For this review, take the finished solid that the model builds, in its own axes (mm). Give positions to 0.01 mm unless a question says otherwise; leave off trailing zeros. Write each loop counter-clockwise with the first axis right and the second up, starting at its lowest first coordinate (ties: lowest second). Pieces come first, ordered by that corner, then holes. Notation, with made-up numbers: M -21,64.25 L 18,64.25 A22 ccw 18,96.25 Z; hole C 81.25,41 d5. An arc over 180 degrees is marked long. Answer as a JSON object with one key per item and string values. Group by question number.
```python
from build123d import *

# Parameters (mm, degrees)
BOSS_EXTRUDE1_DEPTH    = 5
M2_5_CLEARANCE_HOLE1_D = 2.9


with BuildPart() as part:
    # Sketch1 → Boss-Extrude1 (new body)
    with BuildSketch(Plane.XY):
        with BuildLine():
            Line((5, 25), (5, -25))
            ThreePointArc((5, -25), (0, -30), (-5, -25))
            Line((-5, -25), (-5, 25))
            ThreePointArc((-5, 25), (0, 30), (5, 25))
        make_face()
    extrude(amount=BOSS_EXTRUDE1_DEPTH)

    # M2.5 Clearance Hole1 (through all)
    with Locations(Plane.XY.offset(5)):
        with Locations((0, 25), (0, -25)):
            Hole(M2_5_CLEARANCE_HOLE1_D / 2)


solid = part.part
```
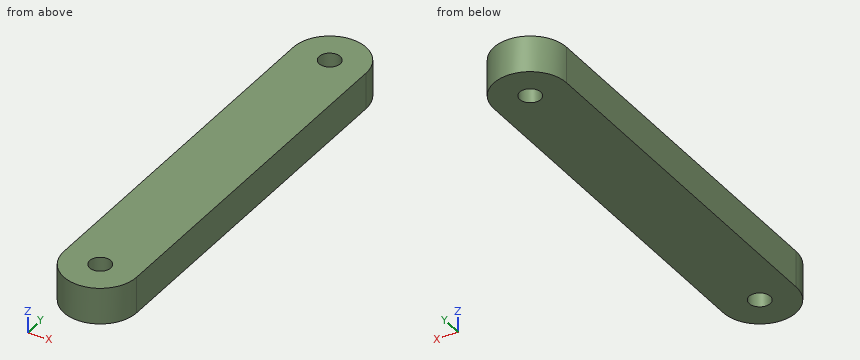
Item 1: Consider section A-A (x = 0). Give the boundary of the cut face in (y, z), plus the area to 3 significant figures.
Item 2: Consider section B-B (z = 2.5). Give the boundary of the cut face in (x, y), plus the area to 3 significant figures.
Item 3: Consider section D-D (x = -2.5). Give the boundary of the cut face in (y, z), plus the area to 3 significant figures.
Item 4: To check wall thickness, follow probe 1 along Y at (x, z) = (0, 1.25); probe 2 along Y at (x, z) = (0.75, 1.35); probe 3 along Y at (x, z) = (3.5, 4.7). State the ranges of each line that lie inside material, in increasing order.
Item 5: Insertion check: P1, Ø3, axis at x = 1, z = 4, coming from the +Y side; P2, Ø2.5, axis at x = 0, y = 25, coming from the +Z side. Each pin has a flat end and moves straight along its axis. Give the tip position at first contact, or say it passes through.
Item 6: Consider section C-C (x = 3.75). Give the boundary of the cut face in (y, z), plus the area to 3 significant figures.
Result set:
{
 "1": {"outline": "M -30,0 L -26.45,0 L -26.45,5 L -30,5 Z; M -23.55,0 L 23.55,0 L 23.55,5 L -23.55,5 Z; M 26.45,0 L 30,0 L 30,5 L 26.45,5 Z", "area": "271 mm^2"},
 "2": {"outline": "M -5,-25 A5 ccw 5,-25 L 5,25 A5 ccw -5,25 Z; hole C 0,-25 d2.9; hole C 0,25 d2.9", "area": "565 mm^2"},
 "3": {"outline": "M -29.33,0 L 29.33,0 L 29.33,5 L -29.33,5 Z", "area": "293 mm^2"},
 "4": {"probe 1": "y = -30 to -26.45, -23.55 to 23.55, 26.45 to 30", "probe 2": "y = -29.94 to -26.24, -23.76 to 23.76, 26.24 to 29.94", "probe 3": "y = -28.57 to 28.57"},
 "5": {"P1": "stops at y = 30", "P2": "passes through"},
 "6": {"outline": "M -28.31,0 L 28.31,0 L 28.31,5 L -28.31,5 Z", "area": "283 mm^2"}
}
